Build history of the part. All positions in model axes, mm. Face numbers are marked on the shaded views. Coordinates: 2 decimals unless noted, no trailing zeros. Loops run counter-clockwise (first coordinate to the right, second up) from the corner with the lowest first, then second, coordinate; pieces in that order, holes last.
(1) Flat gauge pins, fed straight in: P1, Ø1.5, axis at y = 2, z = 35, coming from the +X side; P2, Ø0.9, axis at y = 4.5, z = 28, coming from the +X side; P3, Ø5, axis at y = 4, z = 13.5, coming from the +X side. Where does each tip first touch, or does it go through?
(2) Slice it at A-A (x = 0). Give the cut face in (y, z), and give its area (3 significant figures).
(3) Wall check: L1, parallel to X at y = 0, z = 32.5; L2, parallel to Y at x = 0, z = 13; L3, parallel to X at y = 1, z = 8 (3 decimals). Give the ranges that are in metal, low to high.
(4) Two-plate mould, pull along Y, no slides. Class the marked faces 1, 2 and 3: pulls with the +Y half, pulls with the -Y half, needs draft (parallel to the pull), parting line crosses it, or undercut.
(5) Slice it at C-C (y = -3.5). Give the cut face in (x, z).
(6) Slice it at B-B (z = 29.5). Give the cut face in (x, y), and give its area (3 significant figures).
from build123d import *

# Parameters (mm, degrees)
BOSS_EXTRUDE1_DEPTH = 50
CUT_EXTRUDE1_DEPTH  = 51


with BuildPart() as part:
    # Sketch1 → Boss-Extrude1 (new body)
    with BuildSketch(Plane.XY):
        Polygon((7.332348419, 0), (3.666174209, 6.35), (-3.666174209, 6.35), (-7.332348419, 0), (-3.666174209, -6.35), (3.666174209, -6.35), align=None)
    extrude(amount=BOSS_EXTRUDE1_DEPTH)

    # Sketch2 → Cut-Extrude1 (cut, through all)
    with BuildSketch(Plane.XY.offset(50)):
        with BuildLine():
            Line((-1.048881406, 3.963565036), (-1.048881406, 5.062972332))
            Line((-1.048881406, 5.062972332), (1.051118594, 5.062972332))
            Line((1.051118594, 5.062972332), (1.051118594, 3.962972332))
            ThreePointArc((1.051118594, 3.962972332), (-0.001157185, -4.099999837), (-1.048881406, 3.963565036))
        make_face()
    extrude(amount=-CUT_EXTRUDE1_DEPTH, mode=Mode.SUBTRACT)


solid = part.part
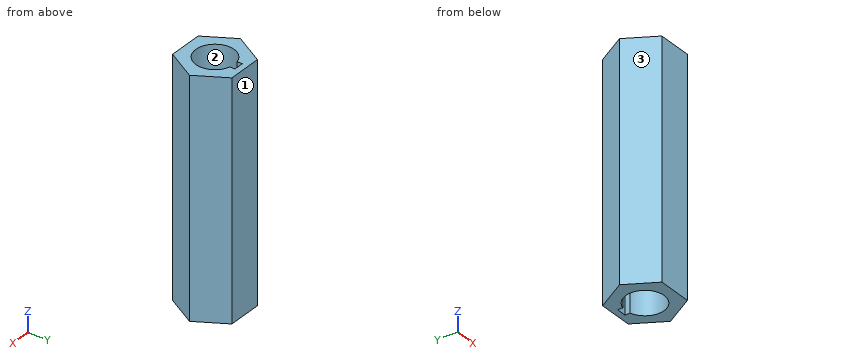
Response values:
1. P1: stops at x = 6.61
1. P2: stops at x = 4.99
1. P3: stops at x = 6.47
2. outline: (-6.35, 0) - (-4.1, 0) - (-4.1, 50) - (-6.35, 50) - close; (5.06, 0) - (6.35, 0) - (6.35, 50) - (5.06, 50) - close
2. area: 177 mm2
3. L1: x = -7.33 to -4.1, 4.1 to 7.33
3. L2: y = -6.35 to -4.1, 5.06 to 6.35
3. L3: x = -6.755 to -3.976, 3.976 to 6.755
4. face 1: pulls with the +Y half
4. face 2: undercut
4. face 3: pulls with the -Y half
5. outline: (-5.31, 0) - (-2.14, 0) - (-2.14, 50) - (-5.31, 50) - close; (2.14, 0) - (5.31, 0) - (5.31, 50) - (2.14, 50) - close
6. outline: (-7.33, 0) - (-3.67, -6.35) - (3.67, -6.35) - (7.33, 0) - (3.67, 6.35) - (-3.67, 6.35) - close; hole (-1.05, 3.96) arc R4.1 ccw (long way) to (1.05, 3.96) - (1.05, 5.06) - (-1.05, 5.06) - close
6. area: 84.8 mm2
